from build123d import *

# Parameters (mm, degrees)
SKETCH1_R           = 2
SKETCH1_R_2         = 5
SKETCH1_R_3         = 4
BOSS_EXTRUDE1_DEPTH = 6


with BuildPart() as part:
    # Sketch1 → Boss-Extrude1 (new body)
    with BuildSketch(Plane.XY):
        with BuildLine():
            Line((-91.133667709, 81.856650449), (-59.395664216, 82.872754588))
            ThreePointArc((-59.395664216, 82.872754588), (-54.441095215, 84.371809376), (-50.89983999, 88.147313406))
            Line((-50.89983999, 88.147313406), (49.994476852, 276.580618392))
            Line((49.994476852, 276.580618392), (30.200235155, 308.463550017))
            ThreePointArc((30.200235155, 308.463550017), (26.424731126, 312.004805242), (21.384421112, 313.183870214))
            Line((21.384421112, 313.183870214), (-16.124128471, 311.983019868))
            Line((-16.124128471, 311.983019868), (-117.018445312, 123.549714881))
            ThreePointArc((-117.018445312, 123.549714881), (-118.197510284, 118.509404867), (-116.698455495, 113.554835867))
            Line((-116.698455495, 113.554835867), (-99.949481752, 86.576970646))
            ThreePointArc((-99.949481752, 86.576970646), (-96.173977723, 83.035715421), (-91.133667709, 81.856650449))
        make_face()
        with Locations((11.628148729, 230.348497445)):
            Circle(SKETCH1_R, mode=Mode.SUBTRACT)
        with Locations((1.104829999, 270.012836125)):
            Circle(SKETCH1_R_2, mode=Mode.SUBTRACT)
        with Locations((-33.33250289, 254.422130449)):
            Circle(SKETCH1_R, mode=Mode.SUBTRACT)
        with Locations((-28.022540924, 156.295659484)):
            Circle(SKETCH1_R, mode=Mode.SUBTRACT)
        with Locations((-72.983192543, 180.369292488)):
            Circle(SKETCH1_R, mode=Mode.SUBTRACT)
        with Locations((-76.464627777, 119.845498823)):
            Circle(SKETCH1_R_3, mode=Mode.SUBTRACT)
    extrude(amount=BOSS_EXTRUDE1_DEPTH)


solid = part.part
Source: CAD feature listing. Evaluate the final solid. Frame: model axes, mm. Round coordinates to 2 decimals unless told otherwise and drop trailing zeros. Write each loop counter-clockwise with the first axis right and the second up, starting at its lowest first coordinate (ties: lowest second). Pieces come first, ordered by that corner, then holes. Notation, with made-up numbers: M 52,-36.5 L 109,-36.5 A19 ccw 109,-9.5 Z; hole C -26.5,43 d8. An arc over 180 degrees is marked long. One line per item, written item: value. Start each with the question number.
Item 1: Section query B-B (x = 36.5). Return the cut outline in (y, z).
Item 2: Pin query (flat end, axial travel): pin 1 (2 mm diameter, centred on x = -8, z = 4.5, fed in from -Y). Return the tip coordinate at first contact, or that it passes through.
Item 3: Section query A-A (z = 4.2). Return the cut outline in (x, y).
Item 4: Section query C-C (y = 291). Return the cut outline in (x, z), plus the area to 3 significant figures.
Item 5: Ray query, L1, parallel to Y at x = 4, z = 5.5; L2, parallel to X at y = 272, z = 0.8; L3, parallel to Y at x = 4.5, z = 0.4. Return the intervals inside material, ascending. Write a range as from..to.
Result set:
1. outline: M 251.38,0 L 298.32,0 L 298.32,6 L 251.38,6 Z
2. pin 1: stops at y = 166.4
3. outline: M -117.02,123.55 A10 ccw -116.7,113.55 L -99.95,86.58 A10 ccw -91.13,81.86 L -59.4,82.87 A10 ccw -50.9,88.15 L 49.99,276.58 L 30.2,308.46 A10 ccw 21.38,313.18 L -16.12,311.98 Z; hole C -76.46,119.85 d8; hole C -72.98,180.37 d4; hole C -33.33,254.42 d4; hole C -28.02,156.3 d4; hole C 1.1,270.01 d10; hole C 11.63,230.35 d4
4. outline: M -27.36,0 L 41.04,0 L 41.04,6 L -27.36,6 Z
4. area: 410 mm²
5. L1: y = 190.68..265.94, 274.09..312.63
5. L2: x = -37.53..-3.48, 5.69..47.54
5. L3: y = 191.61..266.34, 273.68..312.64
